Read the model definition and answer for the solid it produces. Units are mm, in the model's axes. A direction names the side the tool comes from. Give positions to 0.01 mm unless a question says otherwise; leave off trailing zeros. Loops run counter-clockwise (first coordinate to the right, second up) from the corner with the lowest first, then second, coordinate; pieces in that order, holes last. Notation, with made-up numbers: (57, 76.5) - (111, 76.5) arc R17 cw to (111, 83.5) - close; hole circle Ø11 at (-5, 29.25). An arc over 180 degrees is marked (long way). Put each result on its own line as item: value. Start each with the question number.
1. A cutting plane is placed at B-B, the plane y = 28. Determine the outline of the cut face in (x, z), plus the area to 3 significant figures.
2. A cutting plane is placed at C-C, the plane x = -47.5. Determine the outline of the cut face in (y, z), plus the area to 3 significant figures.
3. A cutting plane is placed at A-A, the plane x = -27. Determine the outline of the cut face in (y, z).
4. For faces 5 (the flat face through (-41, 0, -11)), 6 (the flat face through (53, 15.1, -13)), 7 (the cylindrical face through (-54.857, 2.465, 3.965)), determine the directions among +Z, -Z, +X, -X, +Y, -Y from which every point of the face is accessible in a straight line to the end or side of a thin tool.
5. For a pull along X with two mould halves and no side action, classify faces 1 (the cylindrical face through (-14.763, 29.605, 14.302)), 2 (the cylindrical face through (31.24, 29.1, -6.94)), 3 (the cylindrical face through (-11.738, 20.162, 15.844)), 4 (the flat face through (-49, 0, 26)) as released by +X, released by -X, zero draft, split by the parting line, or undercut.
6. Given pin 1 Ø1.5 at (x, z) = (-36.99, -13.94) entering from +Y; pin 2 Ø4.5 at (x, z) = (-15.99, -14.98) entering from -Y; pin 3 Ø2 at (y, z) = (18, 20) entering from -X, each flat-ended and moving along its own axis, determine where each tip first touches the part or whether it passes through.
7. Consider L1, parallel to Z at x = 45.5, y = 3; L2, parallel to X at y = 28.5, z = -15; L3, parallel to Y at x = 49.5, z = 17. Determine where each line is inside the solid, lowest interval first. Write a range as from..to.
```python
from build123d import *

# Parameters (mm, degrees)
SKETCH1_R                                           = 60
BOSS_EXTRUDE1_DEPTH                                 = 36.5
SKETCH2_R                                           = 55
SKETCH2_R_2                                         = 50
CUT_EXTRUDE1_DEPTH                                  = 5
SKETCH5_W                                           = 18
SKETCH5_H                                           = 17
CBORE_FOR_M6_HEX_SOCKET_HEAD_CAP_SCREW1_D           = 6.4
CBORE_FOR_M6_HEX_SOCKET_HEAD_CAP_SCREW1_CBORE_D     = 11
CBORE_FOR_M6_HEX_SOCKET_HEAD_CAP_SCREW1_CBORE_DEPTH = 21.4
M3_CLEARANCE_HOLE1_D                                = 3.4
CBORE_FOR_M3_HEX_SOCKET_HEAD_CAP_SCREW1_D           = 3.4
CBORE_FOR_M3_HEX_SOCKET_HEAD_CAP_SCREW1_CBORE_D     = 6.5
CBORE_FOR_M3_HEX_SOCKET_HEAD_CAP_SCREW1_CBORE_DEPTH = 5.4
SKETCH12_W                                          = 28
SKETCH12_H                                          = 15
M3_TAPPED_HOLE1_D                                   = 2.5
M3_TAPPED_HOLE1_DEPTH                               = 7.5
M3_TAPPED_HOLE1_TIP                                 = 0.751075774


with BuildPart() as part:
    # Sketch1 → Boss-Extrude1 (new body)
    with BuildSketch(Plane(origin=(0, 0, 0), x_dir=(1, 0, 0), z_dir=(0, 1, 0))):
        with Locations(Location((0, 0, 0), (0, 0, 270))):
            Circle(SKETCH1_R)
    extrude(amount=BOSS_EXTRUDE1_DEPTH)

    # Sketch2 → Cut-Extrude1 (cut)
    with BuildSketch(Plane(origin=(0, 0, 0), x_dir=(-1, 0, 0), z_dir=(0, -1, 0))):
        with Locations(Location((0, 0, 0), (0, 0, 90))):
            Circle(SKETCH2_R)
        with Locations(Location((0, 0, 0), (0, 0, 90))):
            Circle(SKETCH2_R_2, mode=Mode.SUBTRACT)
    extrude(amount=-CUT_EXTRUDE1_DEPTH, mode=Mode.SUBTRACT)

    # Sketch4 → Cut-Revolve1 (revolve, cut)
    with BuildSketch(Plane.XY, mode=Mode.PRIVATE) as cut_revolve1_sk:
        Polygon((42, 0), (42, 9), (32.5, 9), (32.5, 16.5), (29, 16.5), (29, 17.5), (10, 17.5), (10, 30.321453401), (0, 30.321453401), (0, 0), align=None)
    revolve(cut_revolve1_sk.sketch.rotate(Axis((0, 0, 0), (0, 1, 0)), 90), axis=Axis((0, 0, 0), (0, 1, 0)), mode=Mode.SUBTRACT)

    # Sketch5 → Cut-Revolve2 (revolve, cut)
    with BuildSketch(Plane.XY, mode=Mode.PRIVATE) as cut_revolve2_sk:
        with Locations((9, 28)):
            Rectangle(SKETCH5_W, SKETCH5_H)
    revolve(cut_revolve2_sk.sketch.rotate(Axis((0, 36.5, 0), (0, -1, 0)), 270), axis=Axis((0, 36.5, 0), (0, -1, 0)), mode=Mode.SUBTRACT)

    # CBORE for M6 Hex Socket Head Cap Screw1 (through all)
    with Locations(Plane(origin=(0, 36.5, 0), x_dir=(1, 0, 0), z_dir=(0, 1, 0))):
        with Locations((51.124173651, -11.94022062), (50.24494344, 15.221552442)):
            CounterBoreHole(CBORE_FOR_M6_HEX_SOCKET_HEAD_CAP_SCREW1_D / 2, CBORE_FOR_M6_HEX_SOCKET_HEAD_CAP_SCREW1_CBORE_D / 2, CBORE_FOR_M6_HEX_SOCKET_HEAD_CAP_SCREW1_CBORE_DEPTH)

    # M3 Clearance Hole1 (through all)
    with Locations(Plane(origin=(0, 36.5, 0), x_dir=(1, 0, 0), z_dir=(0, 1, 0))):
        with Locations((14.984608584, 15.987169155), (15.987169155, -14.984608584), (-14.984608584, -15.987169155), (-15.987169155, 14.984608584)):
            Hole(M3_CLEARANCE_HOLE1_D / 2)

    # CBORE for M3 Hex Socket Head Cap Screw1 (through all)
    with Locations(Plane(origin=(0, 17.5, 0), x_dir=(-1, 0, 0), z_dir=(0, -1, 0))):
        with Locations((15.987169155, 14.984608584), (-14.984608584, 15.987169155), (-15.987169155, -14.984608584), (14.984608584, -15.987169155)):
            CounterBoreHole(CBORE_FOR_M3_HEX_SOCKET_HEAD_CAP_SCREW1_D / 2, CBORE_FOR_M3_HEX_SOCKET_HEAD_CAP_SCREW1_CBORE_D / 2, CBORE_FOR_M3_HEX_SOCKET_HEAD_CAP_SCREW1_CBORE_DEPTH)

    # Sketch12 → Cut-Revolve3 (revolve, cut)
    with BuildSketch(Plane.XY, mode=Mode.PRIVATE) as cut_revolve3_sk:
        with Locations((-46, 29)):
            Rectangle(SKETCH12_W, SKETCH12_H)
    revolve(cut_revolve3_sk.sketch.rotate(Axis((0, 36.5, 0), (0, -1, 0)), 270), axis=Axis((0, 36.5, 0), (0, -1, 0)), mode=Mode.SUBTRACT)

    # M3 Tapped Hole1
    with Locations(Plane(origin=(0, 21.5, 0), x_dir=(1, 0, 0), z_dir=(0, 1, 0))):
        with Locations((13.936224468, 36.986582332), (-36.986582332, 13.936224468), (-36.007862005, -16.299064354), (16.299064354, -36.007862005)):
            Hole(M3_TAPPED_HOLE1_D / 2, depth=M3_TAPPED_HOLE1_DEPTH)
            with Locations((0, 0, -(M3_TAPPED_HOLE1_DEPTH + M3_TAPPED_HOLE1_TIP / 2))):  # 118° drill point
                Cone(0, M3_TAPPED_HOLE1_D / 2, M3_TAPPED_HOLE1_TIP, mode=Mode.SUBTRACT)


solid = part.part
```
Return value:
1. outline: circle Ø64 at (0, 0); hole circle Ø36 at (0, 0); hole circle Ø3.4 at (-15.99, -14.98); hole circle Ø3.4 at (-14.98, 15.99); hole circle Ø3.4 at (14.98, -15.99); hole circle Ø3.4 at (15.99, 14.98)
1. area: 2,160 mm2
2. outline: (0, -36.66) - (21.5, -36.66) - (21.5, 36.66) - (0, 36.66) - (0, 27.73) - (5, 27.73) - (5, 15.61) - (0, 15.61) - (0, -15.61) - (5, -15.61) - (5, -27.73) - (0, -27.73) - close
2. area: 1,460 mm2
3. outline: (0, -53.58) - (21.5, -53.58) - (21.5, -17.18) - (36.5, -17.18) - (36.5, 17.18) - (21.5, 17.18) - (21.5, 53.58) - (0, 53.58) - (0, 47.92) - (5, 47.92) - (5, 42.08) - (0, 42.08) - (0, 32.17) - (9, 32.17) - (9, 18.09) - (16.5, 18.09) - (16.5, 10.58) - (17.5, 10.58) - (17.5, -10.58) - (16.5, -10.58) - (16.5, -18.09) - (9, -18.09) - (9, -32.17) - (0, -32.17) - (0, -42.08) - (5, -42.08) - (5, -47.92) - (0, -47.92) - close
4. face 5: +Z, -Z, +X, -X, -Y
4. face 6: +Y
4. face 7: -Y
5. face 1: undercut
5. face 2: split by the parting line
5. face 3: undercut
5. face 4: zero draft
6. pin 1: stops at y = 13.7
6. pin 2: stops at y = 22.9
6. pin 3: stops at x = -56.91
7. L1: z = -39.11..-30.9, -20.73..20.73, 30.9..39.11
7. L2: x = -28.27..-17.69, -14.29..-9.95, 9.95..13.6, 16.37..28.27
7. L3: y = 5..15.1
